from build123d import *

# Parameters (mm, degrees)
SKETCH1_W                 = 81
SKETCH1_H                 = 88.55
SKETCH1_R                 = 1.75
SKETCH1_R_2               = 1.65
BOSS_EXTRUDE1_DEPTH       = 4
FILLET3_R                 = 0.8
SKETCH2_W                 = 5
SKETCH2_H                 = 20
BOSS_EXTRUDE2_DEPTH       = 8.8
SKETCH5_W                 = 3.2
SKETCH5_H                 = 6.8
CUT_EXTRUDE1_DEPTH        = 94.320362194
FILLET1_SIZE              = 3
FILLET1_SIZE_2            = 5
FILLET2_R                 = 0.5
FILLET1_OF_MIRROR1_SIZE   = 3
FILLET1_OF_MIRROR1_SIZE_2 = 5
FILLET2_OF_MIRROR1_R      = 0.5


with BuildPart() as part:
    # Sketch1 → Boss-Extrude1 (new body)
    with BuildSketch(Plane(origin=(0, 0, 0), x_dir=(1, 0, 0), z_dir=(0, 1, 0))):
        with Locations((40.5, 44.275)):
            Rectangle(SKETCH1_W, SKETCH1_H)
        with Locations(Location((4, 15, 0), (0, 0, 270))):
            Circle(SKETCH1_R, mode=Mode.SUBTRACT)
        with Locations(Location((13.475, 3, 0), (0, 0, 270))):
            Circle(SKETCH1_R_2, mode=Mode.SUBTRACT)
        with Locations(Location((13.475, 85.55, 0), (0, 0, 270))):
            Circle(SKETCH1_R_2, mode=Mode.SUBTRACT)
        with Locations(Location((77, 15, 0), (0, 0, 90))):
            Circle(SKETCH1_R, mode=Mode.SUBTRACT)
        with Locations(Location((67.525, 3, 0), (0, 0, 90))):
            Circle(SKETCH1_R_2, mode=Mode.SUBTRACT)
        with Locations(Location((67.525, 85.55, 0), (0, 0, 90))):
            Circle(SKETCH1_R_2, mode=Mode.SUBTRACT)
    extrude(amount=BOSS_EXTRUDE1_DEPTH)

    # Fillet3
    fillet3_edges = [part.edges().sort_by_distance(p)[0] for p in [
        (81, 4, -44.275),
        (40.5, 4, -88.55),
        (0, 4, -44.275),
        (40.5, 0, -88.55),
        (81, 0, -44.275),
        (40.5, 0, 0),
        (0, 0, -44.275),
        (0, 2, -88.55),
        (81, 2, -88.55),
        (81, 2, 0),
        (0, 2, 0),
        (40.5, 4, 0),
    ]]
    fillet(fillet3_edges, radius=FILLET3_R)

    # Sketch2 → Boss-Extrude2 (add)
    with BuildSketch(Plane.XZ):
        with Locations((13.25, -35.5)):
            Rectangle(SKETCH2_W, SKETCH2_H)
    boss_extrude2 = extrude(amount=BOSS_EXTRUDE2_DEPTH)

    # Sketch5 → Cut-Extrude1 (cut, through all)
    with BuildSketch(Plane(origin=(0, 0, -45.5), x_dir=(-1, 0, 0), z_dir=(0, 0, -1))):
        with Locations((-12.35, -3.4)):
            Rectangle(SKETCH5_W, SKETCH5_H)
    cut_extrude1 = extrude(amount=-CUT_EXTRUDE1_DEPTH, mode=Mode.SUBTRACT)

    # Fillet1
    # an asymmetric fillet: 5, 3 mm, written as the material it adds along each edge
    with BuildSketch(Plane(origin=(15.75, 0, -25.5), x_dir=(1, 0, 0), z_dir=(0, 0, -1))) as fillet1_piece_1:
        with BuildLine():
            Bezier((FILLET1_SIZE, 0), (0, 0), (0, FILLET1_SIZE_2), weights=[1, 0.707106781, 1])
            Line((0, FILLET1_SIZE_2), (0, 0))
            Line((0, 0), (FILLET1_SIZE, 0))
        make_face()
    extrude(amount=20)

    # Fillet2
    fillet2_edges = [part.edges().sort_by_distance(p)[0] for p in [
        (13.25, -8.8, -25.5),
        (13.25, -8.8, -45.5),
        (10.75, -7.8, -25.5),
        (10.75, -7.8, -45.5),
        (10.75, -6.8, -35.5),
        (13.95, -3.4, -45.5),
        (13.95, -3.4, -25.5),
        (10.75, -8.8, -35.5),
        (15.75, -8.8, -35.5),
    ]]
    fillet(fillet2_edges, radius=FILLET2_R)

    # Mirror1: Boss-Extrude2, Cut-Extrude1 across plane
    add(boss_extrude2.mirror(Plane.ZY.offset(-40.5)))
    add(cut_extrude1.mirror(Plane.ZY.offset(-40.5)), mode=Mode.SUBTRACT)

    # Fillet1 of Mirror1
    # an asymmetric fillet: 5, 3 mm, written as the material it adds along each edge
    with BuildSketch(Plane(origin=(65.25, 0, -25.5), x_dir=(-1, 0, 0), z_dir=(0, 0, -1))) as fillet1_of_mirror1_piece_1:
        with BuildLine():
            Bezier((FILLET1_OF_MIRROR1_SIZE, 0), (0, 0), (0, -FILLET1_OF_MIRROR1_SIZE_2), weights=[1, 0.707106781, 1])
            Line((0, -FILLET1_OF_MIRROR1_SIZE_2), (0, 0))
            Line((0, 0), (FILLET1_OF_MIRROR1_SIZE, 0))
        make_face()
    extrude(amount=20)

    # Fillet2 of Mirror1
    fillet2_of_mirror1_edges = [part.edges().sort_by_distance(p)[0] for p in [
        (67.75, -8.8, -25.5),
        (67.75, -8.8, -45.5),
        (70.25, -7.8, -25.5),
        (70.25, -7.8, -45.5),
        (70.25, -6.8, -35.5),
        (67.05, -3.4, -45.5),
        (67.05, -3.4, -25.5),
        (70.25, -8.8, -35.5),
        (65.25, -8.8, -35.5),
    ]]
    fillet(fillet2_of_mirror1_edges, radius=FILLET2_OF_MIRROR1_R)


solid = part.part
The listing builds one solid part. Answer for the finished solid, in the listing's coordinates (mm). A direction names the side the tool comes from. Give positions to 0.01 mm unless a question says otherwise; leave off trailing zeros. Write each loop counter-clockwise with the first axis right and the second up, starting at its lowest first coordinate (ties: lowest second). Pieces come first, ordered by that corner, then holes. Notation, with made-up numbers: (23, 15) - (43, 15) arc R12 ccw to (43, 19) - close; hole circle Ø6 at (-19, -15.5). An arc over 180 degrees is marked (long way). Use a Markdown table: item, result.
1. Section A-A on x = 4 is taken. Write down the section's boundary in (y, z), plus the area to 3 significant figures.
Values follow:
| item | result |
|---|---|
| outline | (0, -87.75) arc R0.8 ccw to (0.8, -88.55) - (3.2, -88.55) arc R0.8 ccw to (4, -87.75) - (4, -16.75) - (0, -16.75) - close; (0, -13.25) - (4, -13.25) - (4, -0.8) arc R0.8 ccw to (3.2, 0) - (0.8, 0) arc R0.8 ccw to (0, -0.8) - close |
| area | 340 mm² |
2. For a pull along X with two mould halves and no side action, classify faces 6 (the flat face through (15.75, -7, -36)), 7 (the cylindrical face through (67.029, 1.972, -87.124)), 8 (the flat face through (67.05, -3, -36)), 9 (the flat face through (66, -5, -45.5)) as released by +X, released by -X, zero draft, split by the parting line, or undercut.
Values follow:
| item | result |
|---|---|
| face 6 | undercut |
| face 7 | undercut |
| face 8 | released by +X |
| face 9 | zero draft |
3. Section D-D on x = 57.5 is taken. Write down the section's boundary in (y, z).
Values follow:
| item | result |
|---|---|
| outline | (0, -87.75) arc R0.8 ccw to (0.8, -88.55) - (3.2, -88.55) arc R0.8 ccw to (4, -87.75) - (4, -0.8) arc R0.8 ccw to (3.2, 0) - (0.8, 0) arc R0.8 ccw to (0, -0.8) - close |
4. Each of these flat-tipped pins is pushed along its axis until it touches: P1, Ø4, axis at y = -6.5, z = -32, coming from the +X side; P2, Ø4, axis at x = 16.5, y = -5, coming from the -Z side; P3, Ø4.5, axis at x = 13.475, z = -85.55, coming from the -Y side. Where does it stop, or does it pass through?
Values follow:
| item | result |
|---|---|
| P1 | stops at x = 70.25 |
| P2 | stops at z = -45.5 |
| P3 | stops at y = 0 |
5. Section B-B on z = -15 is taken. Write down the section's boundary in (x, y), plus the area to 3 significant figures.
Values follow:
| item | result |
|---|---|
| outline | (0, 0.8) arc R0.8 ccw to (0.8, 0) - (2.25, 0) - (2.25, 4) - (0.8, 4) arc R0.8 ccw to (0, 3.2) - close; (5.75, 0) - (75.25, 0) - (75.25, 4) - (5.75, 4) - close; (78.75, 0) - (80.2, 0) arc R0.8 ccw to (81, 0.8) - (81, 3.2) arc R0.8 ccw to (80.2, 4) - (78.75, 4) - close |
| area | 295 mm² |
6. Section C-C on z = -47.5 is taken. Write down the section's boundary in (x, y).
Values follow:
| item | result |
|---|---|
| outline | (0, 0.8) arc R0.8 ccw to (0.8, 0) - (80.2, 0) arc R0.8 ccw to (81, 0.8) - (81, 3.2) arc R0.8 ccw to (80.2, 4) - (0.8, 4) arc R0.8 ccw to (0, 3.2) - close |
7. Find the intervals of material crossed by probe 1 along X at (y, z) = (2.1, -15); probe 2 along X at (y, z) = (1.15, -3) (3 decimals); probe 3 along Y at (x, z) = (13.5, -38), in increasing order. Write a range as from..to.
Values follow:
| item | result |
|---|---|
| probe 1 | x = 0..2.25, 5.75..75.25, 78.75..81 |
| probe 2 | x = 0..11.825, 15.125..65.875, 69.175..81 |
| probe 3 | y = -8.8..-6.8, 0..4 |
8. A tool of negligible diameter and unlimited length cuts with its end or side. For faces 1 (the cylindrical face through (65.89, 1.97, -2.79)), 2 (the flat face through (66, -5, -25.5)), 3 (the flat face through (13.95, -3, -36)), 4 (the flat face through (81, 2, -44)), 5 (the flat face through (15, -4, -45.5)), from which of +Z, -Z, +X, -X, +Y, -Y can it reach the whole face along a straight path? Write none if from no direction.
Values follow:
| item | result |
|---|---|
| face 1 | +Y, -Y |
| face 2 | +Z, +X, -X, -Y |
| face 3 | +Z, -Z, -X |
| face 4 | +Z, -Z, +X, +Y, -Y |
| face 5 | -Z, +X, -X, -Y |
